Work out the finished part from the listing and answer in its coordinate system (mm). A direction names the side the tool comes from. Round coordinates to 2 decimals unless told otherwise and drop trailing zeros. Order: outer loops, then holes, each group sorted by start corner. A loop starts at its lowest first (then second) coordinate and runs counter-clockwise, first axis right, second up.
from build123d import *

# Parameters (mm, degrees)
SKETCH1_R               = 19.25
SKETCH1_R_2             = 4
BOSS_EXTRUDE1_DEPTH     = 4
SKETCH1_4_R             = 4
BOSS_EXTRUDE2_DEPTH     = 27.15
CUT_EXTRUDE1_START      = -1.932
SKETCH6_R               = 4
SKETCH6_R_2             = 3.356
CUT_EXTRUDE1_DEPTH      = 1.932
SKETCH8_R               = 2.5
CUT_EXTRUDE3_DEPTH      = 5
CHAMFER1_SIZE           = 2
CHAMFER1_SIZE2          = 0.727940469
SKETCH9_W               = 0.25
SKETCH9_H               = 2.75
CHAMFER3_SIZE           = 0.3
CHAMFER3_SIZE_2         = 0.210062261
FILLET3_SIZE            = 10
FILLET3_SIZE_2          = 7.5
CUT_EXTRUDE2_DEPTH      = 36.735801376
CUT_EXTRUDE2_DEPTH_BACK = 36.735801376
SKETCH7_R               = 2.25


with BuildPart() as part:
    # Sketch1 → Boss-Extrude1 (new body)
    # profile 1 of 2: a face of its own
    with BuildSketch(Plane(origin=(0, 0, 0), x_dir=(1, 0, 0), z_dir=(0, 1, 0))):
        with Locations(Location((0, 0, 0), (0, 0, 270))):
            Circle(SKETCH1_R)
        with BuildLine():
            ThreePointArc((2, -16.5), (0, -18.5), (-2, -16.5))
            Line((-2, -16.5), (-2, -16.378339354))
            ThreePointArc((-2, -16.378339354), (-14.289419162, -8.25), (-15.184057953, 6.45711887))
            Line((-15.184057953, 6.45711887), (-15.289419162, 6.517949192))
            ThreePointArc((-15.289419162, 6.517949192), (-16.02146997, 9.25), (-13.289419162, 9.982050808))
            Line((-13.289419162, 9.982050808), (-13.184057953, 9.921220485))
            ThreePointArc((-13.184057953, 9.921220485), (0, 16.5), (13.184057953, 9.921220485))
            Line((13.184057953, 9.921220485), (13.289419162, 9.982050808))
            ThreePointArc((13.289419162, 9.982050808), (16.02146997, 9.25), (15.289419162, 6.517949192))
            Line((15.289419162, 6.517949192), (15.184057953, 6.45711887))
            ThreePointArc((15.184057953, 6.45711887), (16.167667677, 3.294923655), (16.5, 0))
            ThreePointArc((16.5, 0), (12.354149101, -10.937321427), (2, -16.378339354))
            Line((2, -16.378339354), (2, -16.5))
        make_face(mode=Mode.SUBTRACT)
    # profile 2 of 2: a face of its own
    with BuildSketch(Plane(origin=(0, 0, 0), x_dir=(1, 0, 0), z_dir=(0, 1, 0))):
        with BuildLine():
            ThreePointArc((-15.184057953, 6.45711887), (-14.289419162, -8.25), (-2, -16.378339354))
            Line((-2, -16.378339354), (-2, -13.96))
            ThreePointArc((-2, -13.96), (0, -11.96), (2, -13.96))
            Line((2, -13.96), (2, -16.378339354))
            ThreePointArc((2, -16.378339354), (12.354149101, -10.937321427), (16.5, 0))
            ThreePointArc((16.5, 0), (16.167667677, 3.294923655), (15.184057953, 6.45711887))
            Line((15.184057953, 6.45711887), (13.089714637, 5.247949192))
            ThreePointArc((13.089714637, 5.247949192), (10.357663829, 5.98), (11.089714637, 8.712050808))
            Line((11.089714637, 8.712050808), (13.184057953, 9.921220485))
            ThreePointArc((13.184057953, 9.921220485), (0, 16.5), (-13.184057953, 9.921220485))
            Line((-13.184057953, 9.921220485), (-11.094979939, 8.715090731))
            Line((-11.094979939, 8.715090731), (-11.089714637, 8.712050808))
            ThreePointArc((-11.089714637, 8.712050808), (-10.357663829, 5.98), (-13.089714637, 5.247949192))
            Line((-13.089714637, 5.247949192), (-15.184057953, 6.45711887))
        make_face()
        with Locations(Location((0, 0, 0), (0, 0, 270))):
            Circle(SKETCH1_R_2, mode=Mode.SUBTRACT)
    extrude(amount=-BOSS_EXTRUDE1_DEPTH)

    # Sketch1<4> → Boss-Extrude2 (add)
    with BuildSketch(Plane(origin=(0, 0, 0), x_dir=(1, 0, 0), z_dir=(0, 1, 0))):
        with Locations(Location((0, 0, 0), (0, 0, 270))):
            Circle(SKETCH1_4_R)
    extrude(amount=-BOSS_EXTRUDE2_DEPTH)

    # Sketch2 → Cut-Revolve4 (revolve, cut)
    with BuildSketch(Plane(origin=(0, 0, 0), x_dir=(0, 0, -1), z_dir=(1, 0, 0)), mode=Mode.PRIVATE) as cut_revolve4_sk:
        Polygon((0, -27.15), (0.8, -27.15), (0.8, -25.15), (1, 0), (0, 0), align=None)
    revolve(cut_revolve4_sk.sketch.rotate(Axis((0, 0, 0), (0, -1, 0)), 180), axis=Axis((0, 0, 0), (0, -1, 0)), mode=Mode.SUBTRACT)

    # Sketch5 → Cut-Revolve8 (revolve, cut)
    with BuildSketch(Plane.XY, mode=Mode.PRIVATE) as cut_revolve8_sk:
        Polygon((0, -7), (-2.55, -5.527756814), (-2.55, 0), (0, 0), align=None)
    revolve(cut_revolve8_sk.sketch.rotate(Axis((0, 0, 0), (0, -1, 0)), 270), axis=Axis((0, 0, 0), (0, -1, 0)), mode=Mode.SUBTRACT)

    # Sketch6 → Cut-Extrude1 (cut)
    with BuildSketch(Plane.XZ.offset(27.15).offset(CUT_EXTRUDE1_START)):
        with Locations(Location((0, 0, 0), (0, 0, 90))):
            Circle(SKETCH6_R)
        with Locations(Location((0, 0, 0), (0, 0, 270))):
            Circle(SKETCH6_R_2, mode=Mode.SUBTRACT)
    extrude(amount=CUT_EXTRUDE1_DEPTH, mode=Mode.SUBTRACT)

    # Sketch8 → Cut-Extrude3 (cut)
    with BuildSketch(Plane(origin=(0, -23, 0), x_dir=(1, 0, 0), z_dir=(0, 1, 0))):
        with Locations((0, 4)):
            Circle(SKETCH8_R)
    extrude(amount=CUT_EXTRUDE3_DEPTH, mode=Mode.SUBTRACT)

    # Chamfer1
    chamfer1_edges = [part.edges().sort_by_distance(p)[0] for p in [
        (0, -18, -4),
    ]]
    chamfer1_side = [part.faces().sort_by_distance(p)[0] for p in [
        (0, -14.609, -4),
    ]]
    chamfer(chamfer1_edges, length=CHAMFER1_SIZE, length2=CHAMFER1_SIZE2, reference=chamfer1_side[0])

    # Sketch9 → Cut-Revolve9 (revolve, cut)
    with BuildSketch(Plane(origin=(0, 0, 0), x_dir=(0, 0, -1), z_dir=(1, 0, 0)), mode=Mode.PRIVATE) as cut_revolve9_sk:
        with Locations((-3.875, -20.5)):
            Rectangle(SKETCH9_W, SKETCH9_H)
    revolve(cut_revolve9_sk.sketch.rotate(Axis((0, -27.15, 0), (0, 1, 0)), 143.580086271), axis=Axis((0, -27.15, 0), (0, 1, 0)), mode=Mode.SUBTRACT)

    # Chamfer3
    # the kernel refuses this chamfer: 0.3, 0.210062261 mm, written as the material it takes off along each edge
    with BuildSketch(Plane(origin=(0, -21.875, 0), x_dir=(-0.42752924874280274, 0, -0.9040015162981834), z_dir=(0.9040015162981834, 0, -0.42752924874280274))) as chamfer3_piece_1_section:
        Polygon((4 - CHAMFER3_SIZE, 0), (4, -CHAMFER3_SIZE_2 * 1.0000000022), (4, 0), align=None)
    chamfer3_piece_1 = revolve(axis=Axis((0, -21.875, 0), (0, 1, 0)), revolution_arc=154.689138052, mode=Mode.PRIVATE)
    chamfer3_piece_1 = chamfer3_piece_1 - Plane(origin=(0, -21.995167344, 0), x_dir=(0.593698599754949, 0, -0.8046874999955033), z_dir=(0, -1, 0)) * Cylinder(3.75, 16, mode=Mode.PRIVATE)
    add(chamfer3_piece_1, mode=Mode.SUBTRACT)
    with BuildSketch(Plane(origin=(0, -21.875, 0), x_dir=(0, 0, 1), z_dir=(-1, 0, 0))) as chamfer3_piece_2_section:
        Polygon((4 - CHAMFER3_SIZE, 0), (4, -CHAMFER3_SIZE_2 * 1.0000000022), (4, 0), align=None)
    chamfer3_piece_2 = revolve(axis=Axis((0, -21.875, 0), (0, 1, 0)), revolution_arc=154.689138052, mode=Mode.PRIVATE)
    chamfer3_piece_2 = chamfer3_piece_2 - Plane(origin=(0, -21.995167344, 0), x_dir=(0.593698599754949, 0, -0.8046874999955033), z_dir=(0, -1, 0)) * Cylinder(3.75, 16, mode=Mode.PRIVATE)
    add(chamfer3_piece_2, mode=Mode.SUBTRACT)

    # Fillet3
    # an asymmetric fillet: 10, 7.5 mm, written as the material it adds along each edge
    with BuildSketch(Plane(origin=(0, -4, 0), x_dir=(0, 0, 1), z_dir=(-1, 0, 0))) as fillet3_piece_1:
        with BuildLine():
            Bezier((4, -FILLET3_SIZE), (4, 0), (4 + FILLET3_SIZE_2, 0), weights=[1, 0.707106781, 1])
            Line((4 + FILLET3_SIZE_2, 0), (4, 0))
            Line((4, 0), (4, -FILLET3_SIZE))
        make_face()
    revolve(axis=Axis((0, -4, 0), (0, 1, 0)))

    # Sketch7 → Cut-Extrude2 (cut, two sides: drawn at the far end of the back side and taken through both)
    with BuildSketch(Plane.XZ.offset(4).offset(-CUT_EXTRUDE2_DEPTH_BACK)):
        with Locations(Location((0, -6.25, 0), (0, 0, 270))):
            Circle(SKETCH7_R)
    extrude(amount=CUT_EXTRUDE2_DEPTH + CUT_EXTRUDE2_DEPTH_BACK, mode=Mode.SUBTRACT)


solid = part.part
Item 1: Find section B-B (z = -12). Write down the section's boundary in (x, y), plus the area to 3 significant figures.
Item 2: Given pin 1 (10 mm diameter, centred on x = 12.5, y = -8.5, fed in from +Z); pin 2 (2 mm diameter, centred on x = 0, z = 0, fed in from +Y); pin 3 (2 mm diameter, centred on y = -1.5, z = 15, fed in from -X), each flat-ended and moving along its own axis, determine where each tip first touches the part or whether it passes through.
Item 3: A tool of negligible diameter and unlimited length cuts with its end or side. For faces 4 (the face through (0, -23, -3)), 5 (the face through (-2, -2, 15)), 6 (the face through (-0.136, -21.999, 3.874)), 7 (the face through (-3, -25.218, -2)), from which of +Z, -Z, +X, -X, +Y, -Y can it reach the whole face along a straight path? Write none if from no direction.
Item 4: For a pull along Z with two mould halves and no side action, classify faces 1 (the face through (3.327, -26.17, 0.437)), 2 (the face through (-1, -27.15, 1)), 3 (the face through (-10.336, -1.972, -6.018)) as released by +Z, released by -Z, zero draft, split by the parting line, or undercut.
Item 5: Find the intervals of material crossed by line 1 along X through (y, z) = (-3.5, -6.25); line 2 along X through (y, z) = (-26.15, 0); line 3 along Y through (x, z) = (-16.5, 0.5), in increasing order.
Item 6: Find section C-C (y = -21). Write down the section's boundary in (x, z), plus the area to 3 significant figures.
Item 7: Find section A-A (x = -14). Write down the section's boundary in (y, z), plus the area to 3 significant figures.
Model answer:
1. outline: (-15.05, -4) - (15.05, -4) - (15.05, 0) - (-15.05, 0) - close
1. area: 120 mm2
2. pin 1: stops at z = 16.25
2. pin 2: stops at y = -6.42
2. pin 3: stops at x = -13.21
3. face 4: -Z
3. face 5: +Y, -Y
3. face 6: none
3. face 7: -Y
4. face 1: split by the parting line
4. face 2: zero draft
4. face 3: undercut
5. line 1: x = -18.21 to -14.83, -10.23 to -2.25, 2.25 to 10.23, 14.83 to 18.21
5. line 2: x = -3.36 to -0.8, 0.8 to 3.36
5. line 3: y = -4 to 0
6. outline: (-2.28, -2.98) arc R2.5 cw to (2.28, -2.98) arc R3.75 ccw (long way) to start; hole circle Ø1.67 at (0, 0)
6. area: 34.7 mm2
7. outline: (-4, -13.21) - (0, -13.21) - (0, -10.23) - (-4, -10.23) - close; (-4, -5.77) - (0, -5.77) - (0, 13.21) - (-4, 13.21) - close
7. area: 87.9 mm2
